Model file for the job. Use its own axes, mm. A direction names the side the tool comes from. Round coordinates to 2 decimals unless told otherwise and drop trailing zeros. Loops run counter-clockwise (first coordinate to the right, second up) from the corner with the lowest first, then second, coordinate; pieces in that order, holes last. Notation, with made-up numbers: M 0,21.5 L 16,21.5 A16 cw 16,42.5 Z; hole C 27.25,-30.75 d2. An arc over 180 degrees is marked long. Use a Markdown table: item, result. Add a question column.
Q1. Probe line 1 (X direction, y = -7.5, z = 1.45); line 2 (X direction, y = -1, z = -0.2); line 3 (Z direction, x = 3, y = -11.5). List the from-to ranges inside material, lowest first. Write a range as from..to.
Q2. Cut at D-D (x = 5). Give the cut face in (y, z).
Q3. Cut at C-C (z = 0.9). Give the cut face in (x, y).
Q4. Cut at A-A (x = 0). Give the cut face in (y, z).
Q5. Mould opens along X. For faces 5 (the face through (-5.6, -4, 0)), 6 (the face through (3.8, -4, -1)), 7 (the face through (-3, -4, 0)) say: +X half, -X half, draft (parallel to the pull), parting line (faces both ways), or undercut.
Q6. Tool access for faces 1 (the face through (-3.8, -4, -1)), 2 (the face through (-0.1, 3.8, -1.3)), 3 (the face through (3.8, -4, 1)), 4 (the face through (-0.1, 3.8, 1.3)): list every direction of +Z, -Z, +X, -X, +Y, -Y with a clear straight run to the whole face (end or side of a thin tool).
Q7. Pin check, flat tips, straight feed: pin 1 (1.1 mm diameter, centred on y = -3, z = 1.5, fed in from -X); pin 2 (3 mm diameter, centred on x = 2, y = -9.5, fed in from +Z); pin 3 (0.7 mm diameter, centred on y = -3, z = -1, fed in from +X). Stop position of each tip, or through.
Q8. Cut at B-B (y = -2.5). Give the cut face in (x, z).
from build123d import *

# Parameters (mm, degrees)
BOSS_EXTRUDE1_DEPTH      = 0.6
BOSS_EXTRUDE1_DEPTH_BACK = 0.6
BOSS_EXTRUDE2_DEPTH      = 2
BOSS_EXTRUDE2_DEPTH_BACK = 2
CUT_EXTRUDE1_DEPTH       = 15.660150067
CUT_EXTRUDE1_DEPTH_BACK  = 15.660150067


with BuildPart() as part:
    # Sketch1 → Boss-Extrude1 (new, two sides: drawn at the far end of the back side and taken through both)
    with BuildSketch(Plane.XY.offset(-BOSS_EXTRUDE1_DEPTH_BACK)):
        with BuildLine():
            Line((5.6, 0), (5.6, -7.8))
            ThreePointArc((5.6, -7.8), (0, -13.4), (-5.6, -7.8))
            Line((-5.6, -7.8), (-5.6, 0))
            ThreePointArc((-5.6, 0), (0, 5.6), (5.6, 0))
        make_face()
        with BuildLine():
            Line((3, 0), (3, -7.8))
            ThreePointArc((3, -7.8), (0, -10.8), (-3, -7.8))
            Line((-3, -7.8), (-3, 0))
            ThreePointArc((-3, 0), (0, 3), (3, 0))
        make_face(mode=Mode.SUBTRACT)
    extrude(amount=BOSS_EXTRUDE1_DEPTH + BOSS_EXTRUDE1_DEPTH_BACK)

    # Sketch1_3 → Boss-Extrude2 (add, two sides: drawn at the far end of the back side and taken through both)
    with BuildSketch(Plane.XY.offset(-BOSS_EXTRUDE2_DEPTH_BACK)):
        with BuildLine():
            Line((3.8, 0), (3.8, -7.8))
            ThreePointArc((3.8, -7.8), (0, -11.6), (-3.8, -7.8))
            Line((-3.8, -7.8), (-3.8, 0))
            ThreePointArc((-3.8, 0), (0, 3.8), (3.8, 0))
        make_face()
    extrude(amount=BOSS_EXTRUDE2_DEPTH + BOSS_EXTRUDE2_DEPTH_BACK)

    # Sketch1_4 → Cut-Extrude1 (cut, two sides: drawn at the far end of the back side and taken through both)
    with BuildSketch(Plane.XY.offset(-CUT_EXTRUDE1_DEPTH_BACK)):
        with BuildLine():
            Line((3, 0), (3, -7.8))
            ThreePointArc((3, -7.8), (0, -10.8), (-3, -7.8))
            Line((-3, -7.8), (-3, 0))
            ThreePointArc((-3, 0), (0, 3), (3, 0))
        make_face()
    extrude(amount=CUT_EXTRUDE1_DEPTH + CUT_EXTRUDE1_DEPTH_BACK, mode=Mode.SUBTRACT)


solid = part.part
Checked values:
| question | item | result |
|---|---|---|
| 1 | line 1 | x = -3.8..-3, 3..3.8 |
| 1 | line 2 | x = -5.6..-3, 3..5.6 |
| 1 | line 3 | z = -0.6..0.6 |
| 2 | outline | M -10.32,-0.6 L 2.52,-0.6 L 2.52,0.6 L -10.32,0.6 Z |
| 3 | outline | M -3.8,-7.8 A3.8 ccw 3.8,-7.8 L 3.8,0 A3.8 ccw -3.8,0 Z; hole M -3,-7.8 A3 ccw 3,-7.8 L 3,0 A3 ccw -3,0 Z |
| 4 | outline | M -13.4,-0.6 L -11.6,-0.6 L -11.6,-2 L -10.8,-2 L -10.8,2 L -11.6,2 L -11.6,0.6 L -13.4,0.6 Z; M 3,-2 L 3.8,-2 L 3.8,-0.6 L 5.6,-0.6 L 5.6,0.6 L 3.8,0.6 L 3.8,2 L 3,2 Z |
| 5 | face 5 | -X half |
| 5 | face 6 | +X half |
| 5 | face 7 | undercut |
| 6 | face 1 | -Z, -X, +Y, -Y |
| 6 | face 2 | -Z, +Y |
| 6 | face 3 | +Z, +X, +Y, -Y |
| 6 | face 4 | +Z, +Y |
| 7 | pin 1 | stops at x = -3.8 |
| 7 | pin 2 | stops at z = 2 |
| 7 | pin 3 | stops at x = 3.8 |
| 8 | outline | M -5.6,-0.6 L -3.8,-0.6 L -3.8,-2 L -3,-2 L -3,2 L -3.8,2 L -3.8,0.6 L -5.6,0.6 Z; M 3,-2 L 3.8,-2 L 3.8,-0.6 L 5.6,-0.6 L 5.6,0.6 L 3.8,0.6 L 3.8,2 L 3,2 Z |
